from build123d import *

# Parameters (mm, degrees)
ESBO_O1_R                = 4
RESSALTO_EXTRUS_O1_DEPTH = 10
CORTE_EXTRUS_O1_DEPTH    = 6
CHANFRO3_SIZE            = 0.5
CHANFRO3_SIZE2           = 0.866025404
CHANFRO4_SIZE            = 2


with BuildPart() as part:
    # Esboço1 → Ressalto-extrusão1 (new body)
    with BuildSketch(Plane.XY):
        Circle(ESBO_O1_R)
    extrude(amount=RESSALTO_EXTRUS_O1_DEPTH)

    # Esboço2 → Corte-extrusão1 (cut)
    with BuildSketch(Plane.XY.offset(10)):
        Polygon((-0.105817982, 2.88481124), (-2.55122881, 1.350764559), (-2.445410828, -1.53404668), (0.105817982, -2.88481124), (2.55122881, -1.350764559), (2.445410828, 1.53404668), align=None)
    extrude(amount=-CORTE_EXTRUS_O1_DEPTH, mode=Mode.SUBTRACT)

    # Chanfro3
    chanfro3_edges = [part.edges().sort_by_distance(p)[0] for p in [
        (-4, 0, 10),
    ]]
    chanfro3_side = [part.faces().sort_by_distance(p)[0] for p in [
        (-4, 0, 5),
    ]]
    chamfer(chanfro3_edges, length=CHANFRO3_SIZE, length2=CHANFRO3_SIZE2, reference=chanfro3_side[0])

    # Chanfro4
    chanfro4_edges = [part.edges().sort_by_distance(p)[0] for p in [
        (-4, 0, 0),
    ]]
    chamfer(chanfro4_edges, length=CHANFRO4_SIZE)


solid = part.part
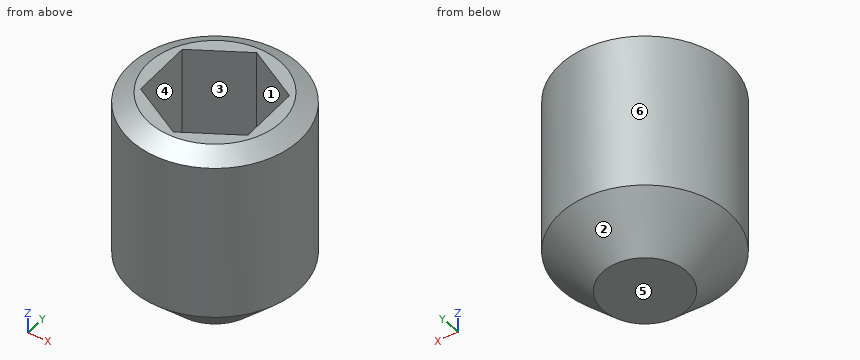
The listing builds one solid part. Answer for the finished solid, in the listing's coordinates (mm). Face numbers are marked on the shaded views. A direction names the side the tool comes from. Give positions to 0.01 mm unless a question says otherwise; leave off trailing zeros. Write each loop counter-clockwise with the first axis right and the second up, starting at its lowest first coordinate (ties: lowest second). Pieces come first, ordered by that corner, then holes.
Item 1: Section A-A, the plane z = 7.5 is taken. Write down the section's boundary in (x, y), plus the area to 3 significant figures.
Item 2: Find the intervals of material crossed by line 1 along X through (y, z) = (-2.5, 9.25); line 2 along X through (y, z) = (1.75, 5.25); line 3 along Y through (x, z) = (-1.75, 9), in increasing order.
Item 3: Determine the mould class of the marked faces 3, 4, 5 and 6 for opening direction Y: released by +Y, released by -Y, zero draft, split by the parting line, or undercut.
Item 4: Section B-B, the plane z = 2.5 is taken. Write down the section's boundary in (x, y).
Item 5: A flat-ended cylindrical pin translates along its axis: P1, Ø2.5, axis at x = 1, y = 1, coming from the +Z side. Find the tip coordinate at first contact, or state that the pin passes through.
Item 6: Which of the six approach directions +Z, -Z, +X, -X, +Y, -Y give full straight-line access (tool end or side, diameter ignored) to the marked faces 1 and 2?
Completed:
1. outline: circle Ø8 at (0, 0); hole (-2.55, 1.35) - (-2.45, -1.53) - (0.11, -2.88) - (2.55, -1.35) - (2.45, 1.53) - (-0.11, 2.88) - close
1. area: 28.6 mm2
2. line 1: x = -3.12 to -0.62, 0.72 to 3.12
2. line 2: x = -3.6 to -1.91, 2.04 to 3.6
2. line 3: y = -3.6 to -1.9, 1.85 to 3.6
3. face 3: undercut
3. face 4: undercut
3. face 5: zero draft
3. face 6: split by the parting line
4. outline: circle Ø8 at (0, 0)
5. P1: stops at z = 10
6. face 1: +Z
6. face 2: -Z
